Could you check a few things on this model? Use its own coordinates, in mm. A direction names the side the tool comes from. Round coordinates to 2 decimals unless told otherwise and drop trailing zeros. Loops run counter-clockwise (first coordinate to the right, second up) from the corner with the lowest first, then second, coordinate; pieces in that order, holes last.
from build123d import *

# Parameters (mm, degrees)
SKETCH1_R           = 1.27
BOSS_EXTRUDE1_DEPTH = 2.5
SKETCH2_W           = 19.957142857
SKETCH2_H           = 2.5
CUT_EXTRUDE1_DEPTH  = 2.5
CUT_EXTRUDE2_DEPTH  = 2.5
SKETCH4_R           = 1.5
CUT_EXTRUDE3_DEPTH  = 2.5
SKETCH5_R           = 7.239
SKETCH5_R_2         = 1.5
CUT_EXTRUDE4_DEPTH  = 2.5
SKETCH6_R           = 4.83219682
SKETCH6_R_2         = 1.5
CUT_EXTRUDE5_DEPTH  = 2.5
SKETCH7_R           = 1.5
CUT_EXTRUDE6_DEPTH  = 2.54
FILLET1_R           = 7.62


with BuildPart() as part:
    # Sketch1 → Boss-Extrude1 (new body)
    with BuildSketch(Plane(origin=(0, 0, 0), x_dir=(1, 0, 0), z_dir=(0, 1, 0))):
        Polygon((0, 0), (-38.1, 0), (-38.1, -55.88), (-18.034, -55.88), (-18.034, -68.58), (1.905, -68.58), (1.905, -55.88), (101.6, -55.88), (174.591014612, 14.794406866), (139.253811179, 51.289914172), (76.2, 0), (50.8, 0), (50.8, 38.374100719), (0, 38.374100719), align=None)
        with Locations(Location((-8.0645, -62.23, 0), (0, 0, 270))):
            Circle(SKETCH1_R, mode=Mode.SUBTRACT)
    extrude(amount=BOSS_EXTRUDE1_DEPTH)

    # Sketch2 → Cut-Extrude1 (cut)
    with BuildSketch(Plane(origin=(0, 2.5, 0), x_dir=(1, 0, 0), z_dir=(0, 1, 0))):
        with Locations((-28.121428572, -54.63)):
            Rectangle(SKETCH2_W, SKETCH2_H)
        with Locations((11.792857143, -54.63)):
            Rectangle(SKETCH2_W, SKETCH2_H)
        with Locations((51.707142858, -54.63)):
            Rectangle(SKETCH2_W, SKETCH2_H)
        with Locations((91.621428572, -54.63)):
            Rectangle(SKETCH2_W, SKETCH2_H)
    extrude(amount=-CUT_EXTRUDE1_DEPTH, mode=Mode.SUBTRACT)

    # Sketch3 → Cut-Extrude2 (cut)
    with BuildSketch(Plane(origin=(0, 2.5, 0), x_dir=(1, 0, 0), z_dir=(0, 1, 0))):
        Polygon((101.685739763, -52.317101083), (103.424775365, -54.113139828), (113.591380972, -44.269204586), (111.85234537, -42.473165841), align=None)
        Polygon((122.018950977, -32.629230599), (123.757986579, -34.425269344), (133.924592185, -24.581334102), (132.185556583, -22.785295357), align=None)
        Polygon((142.35216219, -12.941360115), (144.091197792, -14.73739886), (154.257803399, -4.893463618), (152.518767797, -3.097424873), align=None)
        Polygon((162.685373403, 6.74651037), (164.424409005, 4.950471624), (174.591014612, 14.794406866), (172.85197901, 16.590445612), align=None)
    extrude(amount=-CUT_EXTRUDE2_DEPTH, mode=Mode.SUBTRACT)

    # Sketch4 → Cut-Extrude3 (cut)
    with BuildSketch(Plane(origin=(0, 2.5, 0), x_dir=(1, 0, 0), z_dir=(0, 1, 0))):
        with Locations(Location((-4.285702379, -2.932700938, 0), (0, 0, 270))):
            Circle(SKETCH4_R)
        with Locations(Location((-35.019835528, -2.932700938, 0), (0, 0, 270))):
            Circle(SKETCH4_R)
        with Locations(Location((3.703940689, 34.739752907, 0), (0, 0, 270))):
            Circle(SKETCH4_R)
        with Locations(Location((46.856938601, 34.739752907, 0), (0, 0, 270))):
            Circle(SKETCH4_R)
        with Locations(Location((137.828101929, 46.33680801, 0), (0, 0, 270))):
            Circle(SKETCH4_R)
        with Locations(Location((109.860015666, 23.133232504, 0), (0, 0, 270))):
            Circle(SKETCH4_R)
        with Locations(Location((123.849763227, 34.739752907, 0), (0, 0, 270))):
            Circle(SKETCH4_R)
    extrude(amount=-CUT_EXTRUDE3_DEPTH, mode=Mode.SUBTRACT)

    # Sketch5 → Cut-Extrude4 (cut)
    with BuildSketch(Plane(origin=(0, 2.5, 0), x_dir=(1, 0, 0), z_dir=(0, 1, 0))):
        with Locations(Location((25.4, 10.434100719, 0), (0, 0, 270))):
            Circle(SKETCH5_R)
        with Locations(Location((12.954, 10.434100719, 0), (0, 0, 270))):
            Circle(SKETCH5_R_2)
        with Locations(Location((37.846, 10.434100719, 0), (0, 0, 270))):
            Circle(SKETCH5_R_2)
    extrude(amount=-CUT_EXTRUDE4_DEPTH, mode=Mode.SUBTRACT)

    # Sketch6 → Cut-Extrude5 (cut)
    with BuildSketch(Plane(origin=(0, 2.5, 0), x_dir=(1, 0, 0), z_dir=(0, 1, 0))):
        with Locations(Location((77.47, -5.588, 0), (0, 0, 270))):
            Circle(SKETCH6_R)
        with Locations(Location((69.088, -5.588, 0), (0, 0, 270))):
            Circle(SKETCH6_R_2)
        with Locations(Location((85.852, -5.588, 0), (0, 0, 270))):
            Circle(SKETCH6_R_2)
    extrude(amount=-CUT_EXTRUDE5_DEPTH, mode=Mode.SUBTRACT)

    # Sketch7 → Cut-Extrude6 (cut)
    with BuildSketch(Plane(origin=(0, 2.5, 0), x_dir=(1, 0, 0), z_dir=(0, 1, 0))):
        with Locations(Location((99.525450368, -50.013841017, 0), (0, 0, 270))):
            Circle(SKETCH7_R)
    extrude(amount=-CUT_EXTRUDE6_DEPTH, mode=Mode.SUBTRACT)

    # Fillet1
    fillet1_edges = [part.edges().sort_by_distance(p)[0] for p in [
        (1.905, 1.25, 68.58),
        (-18.034, 1.25, 68.58),
    ]]
    fillet(fillet1_edges, radius=FILLET1_R)


solid = part.part
Item 1: We'd pull the mould along Z, two halves only. Please class faces 1 (the cylindrical face through (18.98, 1.27, -7.09)), 2 (the flat face through (156.288, 1.232, -33.697)), 3 (the flat face through (118.6, 1.23, 39.42)): released by +Z, released by -Z, zero draft, split by the parting line, or undercut.
Results list:
face 1: undercut
face 2: released by -Z
face 3: released by +Z
Item 2: If we section it at C-C, the plane x = 129.5: Please give me the cut outline in (y, z).
Results list:
outline: (0, -43.36) - (2.5, -43.36) - (2.5, 25.39) - (0, 25.39) - close
Item 3: If we section it at D-D, the plane x = 96: Please give me the cut outline in (y, z).
Results list:
outline: (0, -16.11) - (2.5, -16.11) - (2.5, 53.38) - (0, 53.38) - close
Item 4: If I drill on line 1 along X through (y, z) = (1.2, -10.5); line 2 along Z through (x, y) = (54, 1.45); line 3 along X through (y, z) = (0.4, -8.5), over which ranges is the centre line in solid material (lowest first)?
Results list:
line 1: x = 0 to 11.46, 14.45 to 18.16, 32.64 to 36.35, 39.34 to 50.8, 89.11 to 166.56
line 2: z = 0 to 53.38
line 3: x = 0 to 18.42, 32.38 to 50.8, 86.65 to 164.5
Item 5: If we section it at A-A, the plane x = 25.4: Please give me the cut outline in (y, z), then the cut area to 3 significant figures.
Results list:
outline: (0, -38.37) - (2.5, -38.37) - (2.5, -17.67) - (0, -17.67) - close; (0, -3.2) - (2.5, -3.2) - (2.5, 55.88) - (0, 55.88) - close
area: 199 mm2
Item 6: For faces 4 (the cylindrical face through (72.753, 1.268, 4.54)), 5 (the flat face through (108.168, 1.232, -26.004)), which set-ups out of +Z, -Z, +X, -X, +Y, -Y let a thin tool reach every point of the face, with its end or its side?
Results list:
face 4: +Y, -Y
face 5: -Z, +Y, -Y
Item 7: If we section it at B-B, the plane y = 0.95: Count the separate pieces of the cut face and the enclosed holes in it, then the cut area to 3 significant figures.
Results list:
separate pieces: 1
enclosed holes: 15
area: 13,600 mm2
Item 8: Will these pins go through, and if not, where does the flat tip stop? pin 1 (5 mm diameter, centred on x = 69.088, z = 5.588, fed in from +Y); pin 2 (0.8 mm diameter, centred on y = 1, z = 57.5, fed in from +X) (3 decimals); pin 3 (1.2 mm diameter, centred on x = 74, y = 1, fed in from +Z); pin 4 (1.5 mm diameter, centred on y = 1.5, z = 49.5, fed in from +X).
Results list:
pin 1: stops at y = 2.5
pin 2: stops at x = 1.905
pin 3: stops at z = 55.88
pin 4: stops at x = 105.37
